Geometry check sheet. Reference: the model listing, model coordinates, mm. Coordinates: 2 decimals unless noted, no trailing zeros. Order: outer loops, then holes, each group sorted by start corner. A loop starts at its lowest first (then second) coordinate and runs counter-clockwise, first axis right, second up. Notation, with made-up numbers: (40, 70) - (58, 70) arc R16 cw to (58, 96) - close; hole circle Ø7 at (43, -1.5). An arc over 180 degrees is marked (long way). Return JSON: item names as keys, results as strings. Group by question number.
Item 1: Section check B-B on y = 2. Enter the section's corners in (x, z).
Item 2: Section check D-D on x = 4.75. Enter the section's corners in (y, z).
Item 3: Draft check along X on faces 1 (the flat face through (0, -7, -20)), 2 (the cylindrical face through (-3, 0, 0)), 3 (the flat face through (-6, -7, 0)). Enter one of: pulls with the +X half, pulls with the -X half, needs draft (parallel to the pull), parting line crosses it, or undercut.
Item 4: Scan lines: probe 1 along Y at (x, z) = (0, 9); probe 2 along X at (y, z) = (1.75, -7); probe 3 along Y at (x, z) = (-2.5, 7.5). Record each from-to range of solid material in increasing order.
Item 5: Gauge pin test, flat ends, axial feed: pin 1 (1 mm diameter, centred on x = 2, z = -14, fed in from +Y); pin 2 (5 mm diameter, centred on x = 0, y = 0, fed in from +Z). Record the tip position at first contact, or that the pin passes through.
Item 6: Section check C-C on y = -15.5. Enter the section's corners in (x, z), then the cut area to 3 significant figures.
from build123d import *

# Parameters (mm, degrees)
SKETCH1_W           = 12
SKETCH1_H           = 26
SKETCH1_R           = 3
BOSS_EXTRUDE1_DEPTH = 20
FILLET1_R           = 6
FILLET2_R           = 4


with BuildPart() as part:
    # Sketch1 → Boss-Extrude1 (new, symmetric)
    with BuildSketch(Plane.XY):
        with Locations((0, -7)):
            Rectangle(SKETCH1_W, SKETCH1_H)
        Circle(SKETCH1_R, mode=Mode.SUBTRACT)
    extrude(amount=BOSS_EXTRUDE1_DEPTH, both=True)

    # Fillet1
    fillet1_edges = [part.edges().sort_by_distance(p)[0] for p in [
        (-6, -20, 0),
        (6, 6, 0),
        (-6, 6, 0),
    ]]
    fillet(fillet1_edges, radius=FILLET1_R - 0.0001)  # a hair under: the kernel refuses the full size

    # Fillet2
    fillet2_edges = [part.edges().sort_by_distance(p)[0] for p in [
        (6, -20, 0),
    ]]
    fillet(fillet2_edges, radius=FILLET2_R)


solid = part.part
Computed:
{
 "1": {"outline": "(-5.66, -20) - (-2.24, -20) - (-2.24, 20) - (-5.66, 20) - close; (2.24, -20) - (5.66, -20) - (5.66, 20) - (2.24, 20) - close"},
 "2": {"outline": "(-18.9, -20) - (3.67, -20) - (3.67, 20) - (-18.9, 20) - close"},
 "3": {"face 1": "needs draft", "face 2": "undercut", "face 3": "pulls with the -X half"},
 "4": {"probe 1": "y = -20 to -3, 3 to 6", "probe 2": "x = -5.74 to -2.44, 2.44 to 5.74", "probe 3": "y = -19.45 to -1.66, 1.66 to 5.45"},
 "5": {"pin 1": "stops at y = 5.81", "pin 2": "passes through"},
 "6": {"outline": "(-5.81, -20) - (6, -20) - (6, 20) - (-5.81, 20) - close", "area": "472 mm²"}
}
